Input: part model. Units: mm. Frame: model coordinates. A direction names the side the tool comes from. Give positions to 0.01 mm unless a question says otherwise; leave off trailing zeros. Loops run counter-clockwise (first coordinate to the right, second up) from the corner with the lowest first, then second, coordinate; pieces in that order, holes last. Notation, with made-up numbers: M -27,50 L -3,50 A21 ccw -3,55 Z; hole C 36,-15 d10. An arc over 180 degrees is marked long. Answer as a JSON object with one key per item and string values. Group by question number.
```python
from build123d import *

# Parameters (mm, degrees)
SKETCH_1_W           = 112
SKETCH_1_H           = 140
EXTRUDE_1_DEPTH      = 2.5
CUT_EXTRUDE_2_DEPTH  = 5
SKETCH_4_R           = 2.025
CUT_EXTRUDE_3_DEPTH  = 10
SKETCH_6_W           = 18
SKETCH_6_H           = 13
CUT_EXTRUDE_5_DEPTH  = 10
CUT_EXTRUDE_6_DEPTH  = 5
FILLET_1_R           = 3
SKETCH_8_R           = 1.525
CUT_EXTRUDE_7_DEPTH  = 5
SKETCH_10_R          = 2.525
CUT_EXTRUDE_9_DEPTH  = 40
FILLET_3_R           = 3
CUT_EXTRUDE_10_DEPTH = 78
EXTRUDE_2_DEPTH      = 5
EXTRUDE_3_DEPTH      = 5
FILLET_4_R           = 1.5
EXTRUDE_6_DEPTH      = 5
SKETCH_22_R          = 1.525
CUT_EXTRUDE_15_DEPTH = 5
SKETCH_24_R          = 2.025
CUT_EXTRUDE_17_DEPTH = 10


with BuildPart() as part:
    # 草图1 → 凸台-拉伸1 (new, symmetric)
    with BuildSketch(Plane.XY):
        Rectangle(SKETCH_1_W, SKETCH_1_H)
    extrude(amount=EXTRUDE_1_DEPTH, both=True)

    # 草图3 → 切除-拉伸2 (cut)
    with BuildSketch(Plane.XY.offset(2.5)):
        Polygon((-15, 70), (-56, 50), (-56, 70), align=None)
        Polygon((56, 70), (15, 70), (56, 50), align=None)
    extrude(amount=-CUT_EXTRUDE_2_DEPTH, mode=Mode.SUBTRACT)

    # 草图4 → 切除-拉伸3 (cut)
    with BuildSketch(Plane.XY.offset(2.5)):
        with Locations((0, -3.65)):
            Circle(SKETCH_4_R)
        with Locations((43, -3.65)):
            Circle(SKETCH_4_R)
        with Locations((-43, -3.65)):
            Circle(SKETCH_4_R)
        with Locations((-43, 23)):
            Circle(SKETCH_4_R)
        with Locations((0, 42.696305337)):
            Circle(SKETCH_4_R)
        with Locations((43, 23)):
            Circle(SKETCH_4_R)
    extrude(amount=-CUT_EXTRUDE_3_DEPTH, mode=Mode.SUBTRACT)

    # 草图6 → 切除-拉伸5 (cut)
    with BuildSketch(Plane(origin=(0, 0, -2.5), x_dir=(-1, 0, 0), z_dir=(0, 0, -1))):
        with Locations((47, -63.5)):
            Rectangle(SKETCH_6_W, SKETCH_6_H)
    cut_extrude_5 = extrude(amount=-CUT_EXTRUDE_5_DEPTH, mode=Mode.SUBTRACT)

    # 镜向2: 切除-拉伸5 across plane
    add(cut_extrude_5.mirror(Plane(origin=(0, 0, 0), x_dir=(0, 0, 1), z_dir=(1, 0, 0))), mode=Mode.SUBTRACT)

    # 草图7 → 切除-拉伸6 (cut)
    with BuildSketch(Plane.XY.offset(2.5)):
        Polygon((-3, 1.35), (-3, 35.822569262), (-38, 19.790692824), (-38, 1.35), align=None)
        Polygon((38, 19.790692824), (3, 35.822569262), (3, 1.35), (38, 1.35), align=None)
    extrude(amount=-CUT_EXTRUDE_6_DEPTH, mode=Mode.SUBTRACT)

    # 圆角1
    fillet_1_edges = [part.edges().sort_by_distance(p)[0] for p in [
        (-38, 19.790692824, 0),
        (-38, 1.35, 0),
        (-3, 1.35, 0),
        (-3, 35.822569262, 0),
        (3, 1.35, 0),
        (38, 1.35, 0),
        (38, 19.790692824, 0),
        (3, 35.822569262, 0),
    ]]
    fillet(fillet_1_edges, radius=FILLET_1_R)

    # 草图8 → 切除-拉伸7 (cut)
    with BuildSketch(Plane(origin=(0, 0, -2.5), x_dir=(-1, 0, 0), z_dir=(0, 0, -1))):
        with Locations((-53, 2)):
            Circle(SKETCH_8_R)
        with Locations((-53, -18)):
            Circle(SKETCH_8_R)
    cut_extrude_7 = extrude(amount=-CUT_EXTRUDE_7_DEPTH, mode=Mode.SUBTRACT)

    # 镜向3: 切除-拉伸7 across plane
    add(cut_extrude_7.mirror(Plane(origin=(0, 0, 0), x_dir=(0, 0, 1), z_dir=(1, 0, 0))), mode=Mode.SUBTRACT)

    # 草图10 → 切除-拉伸9 (cut)
    with BuildSketch(Plane.XY.offset(2.5)):
        with Locations((-30, -64)):
            Circle(SKETCH_10_R)
        with Locations((30, -64)):
            Circle(SKETCH_10_R)
    extrude(amount=-CUT_EXTRUDE_9_DEPTH, mode=Mode.SUBTRACT)

    # 圆角3
    fillet_3_edges = [part.edges().sort_by_distance(p)[0] for p in [
        (-56, 50, 0),
        (-15, 70, 0),
        (15, 70, 0),
        (56, 50, 0),
        (-56, -57, 0),
        (-38, -70, 0),
        (-38, -57, 0),
        (56, -57, 0),
        (38, -57, 0),
        (38, -70, 0),
    ]]
    fillet(fillet_3_edges, radius=FILLET_3_R)

    # 草图11 → 切除-拉伸10 (cut)
    with BuildSketch(Plane(origin=(0, 0, -2.5), x_dir=(-1, 0, 0), z_dir=(0, 0, -1))):
        Polygon((-6.884052732, -51), (-48, -11.425900755), (-48, -51), align=None)
        Polygon((-4, -8.65), (-45.115947268, -8.65), (-4, -48.224099245), align=None)
    cut_extrude_10 = extrude(amount=-CUT_EXTRUDE_10_DEPTH, mode=Mode.SUBTRACT)

    # 草图12 → 凸台-拉伸2 (add)
    with BuildSketch(Plane(origin=(0, 0, -2.5), x_dir=(-1, 0, 0), z_dir=(0, 0, -1))):
        Polygon((-27.442026366, -8.65), (-4, -31.212950377), (-2.613062807, -26.996075916), (-23.171036441, -7.209026293), align=None)
        Polygon((-49.386937193, -32.653924084), (-28.828963559, -52.440973707), (-24.557973634, -51), (-48, -28.437049623), align=None)
    extrude_2 = extrude(amount=-EXTRUDE_2_DEPTH)

    # 草图13 → 凸台-拉伸3 (add)
    with BuildSketch(Plane(origin=(0, 0, -2.5), x_dir=(-1, 0, 0), z_dir=(0, 0, -1))):
        Polygon((-29.446658669, -8.65), (-26.553352036, -51.135886105), (-22.553341331, -51), (-25.446647964, -8.514113895), align=None)
    extrude_3 = extrude(amount=-EXTRUDE_3_DEPTH)

    # 镜向5: 切除-拉伸10, 凸台-拉伸2, 凸台-拉伸3 across plane
    add(cut_extrude_10.mirror(Plane(origin=(0, 0, 0), x_dir=(0, 0, 1), z_dir=(1, 0, 0))), mode=Mode.SUBTRACT)
    add(extrude_2.mirror(Plane(origin=(0, 0, 0), x_dir=(0, 0, 1), z_dir=(1, 0, 0))))
    add(extrude_3.mirror(Plane(origin=(0, 0, 0), x_dir=(0, 0, 1), z_dir=(1, 0, 0))))

    # 圆角4
    fillet_4_edges = [part.edges().sort_by_distance(p)[0] for p in [
        (4, -48.224099245, 0),
        (45.115947268, -8.65, 0),
        (4, -8.65, 0),
        (6.884052732, -51, 0),
        (48, -51, 0),
        (48, -11.425900755, 0),
        (4, -25.661148868, 0),
        (21.673920902, -8.65, 0),
        (4, -31.212950377, 0),
        (48, -33.988851132, 0),
        (30.326079098, -51, 0),
        (48, -28.437049623, 0),
        (26.703219631, -48.935200727, 0),
        (25.296780369, -10.714799273, 0),
        (23.652453905, -34.860413872, 0),
        (27.942945899, -30.730815326, 0),
        (29.446658669, -8.65, 0),
        (24.057054101, -28.919184674, 0),
        (22.553341331, -51, 0),
        (28.347546095, -24.789586128, 0),
        (-45.115947268, -8.65, 0),
        (-4, -48.224099245, 0),
        (-4, -8.65, 0),
        (-48, -51, 0),
        (-6.884052732, -51, 0),
        (-48, -11.425900755, 0),
        (-21.673920902, -8.65, 0),
        (-4, -25.661148868, 0),
        (-4, -31.212950377, 0),
        (-48, -33.988851132, 0),
        (-30.326079098, -51, 0),
        (-48, -28.437049623, 0),
        (-26.703219631, -48.935200727, 0),
        (-25.296780369, -10.714799273, 0),
        (-23.652453905, -34.860413872, 0),
        (-24.057054101, -28.919184674, 0),
        (-22.553341331, -51, 0),
        (-27.942945899, -30.730815326, 0),
        (-28.347546095, -24.789586128, 0),
        (-29.446658669, -8.65, 0),
    ]]
    fillet(fillet_4_edges, radius=FILLET_4_R)

    # 草图21 → 凸台-拉伸6 (add)
    with BuildSketch(Plane(origin=(0, 0, -2.5), x_dir=(-1, 0, 0), z_dir=(0, 0, -1))):
        with BuildLine():
            Line((-20, -3), (-25.822161429, -3))
            Line((-25.822161429, -3), (-25.413558917, -9))
            Line((-25.413558917, -9), (-20, -9))
            ThreePointArc((-20, -9), (-17, -6), (-20, -3))
        make_face()
    extrude(amount=-EXTRUDE_6_DEPTH)

    # 草图22 → 切除-拉伸15 (cut)
    with BuildSketch(Plane(origin=(0, 0, -2.5), x_dir=(-1, 0, 0), z_dir=(0, 0, -1))):
        with Locations((0, -6)):
            Circle(SKETCH_22_R)
        with Locations((-20, -6)):
            Circle(SKETCH_22_R)
    extrude(amount=-CUT_EXTRUDE_15_DEPTH, mode=Mode.SUBTRACT)

    # 草图24 → 切除-拉伸17 (cut)
    with BuildSketch(Plane.XY.offset(2.5)):
        with Locations((-15, -64)):
            Circle(SKETCH_24_R)
        with Locations((15, -64)):
            Circle(SKETCH_24_R)
    extrude(amount=-CUT_EXTRUDE_17_DEPTH, mode=Mode.SUBTRACT)


solid = part.part
```
1. Material intervals for L1, parallel to X at y = 11.5, z = -0.9; L2, parallel to Y at x = -43, z = 0.65 (3 decimals); L3, parallel to Y at x = 39.5, z = 1, sorted ascending.
2. Mould query, pull axis Y, two halves, no side actions, for faces 3 (the flat face through (12, -8.65, 0)), 4 (the cylindrical face through (55.53, 49.74, -0.04)), 5 (the cylindrical face through (55.14, -56.1, 0.04)). Classes: pulls with the +Y half, pulls with the -Y half, needs draft (parallel to the pull), parting line crosses it, or undercut.
3. Section A-A (y = 6.5). Output: boundary loops of the cut face in (x, z), then the cut area to 3 significant figures.
4. Reachability of faces 1 (the flat face through (-1, 1, -2.5)), 2 (the flat face through (39.321, -42.343, -0.035)) from +Z, -Z, +X, -X, +Y, -Y: full face, straight path, thin tool, end or side. Return the list, or none.
5. Section B-B (y = 23). Output: boundary loops of the cut face in (x, z) (3 decimals).
6. Section D-D (z = 1.45). Count the separate pieces of the cut face and the enclosed holes in it, then the cut area to 3 significant figures.
7. First-contact query: P1, Ø1.5, axis at x = 19, z = 0.5, coming from the +Y side; P2, Ø1.5, axis at x = 39.5, z = -1.5, coming from the -Y side. Flat tips, straight axial feed; report the tip coordinate or a pass-through.
8. Section C-C (y = 53). Output: boundary loops of the cut face in (x, z), then the cut area to 4 significant figures.
Geometry results:
{
 "1": {"L1": "-56 to -38, -3 to 3, 38 to 56", "L2": "-57 to -51, -38.801 to -33.25, -16.238 to -5.675, -1.625 to 20.975, 25.025 to 56.341", "L3": "-57.4 to -51, -42.17 to -36.62, -19.61 to -14.06, -8.65 to 58.05"},
 "2": {"face 3": "undercut", "face 4": "pulls with the +Y half", "face 5": "pulls with the -Y half"},
 "3": {"outline": "M -56,-2.5 L -38,-2.5 L -38,2.5 L -56,2.5 Z; M -3,-2.5 L 3,-2.5 L 3,2.5 L -3,2.5 Z; M 38,-2.5 L 56,-2.5 L 56,2.5 L 38,2.5 Z", "area": "210 mm2"},
 "4": {"face 1": "-Z, +X, -X, +Y, -Y", "face 2": "+Z, -Z"},
 "5": {"outline": "M -56,-2.5 L -45.025,-2.5 L -45.025,2.5 L -56,2.5 Z; M -40.975,-2.5 L -30.994,-2.5 L -30.994,2.5 L -40.975,2.5 Z; M -3,-2.5 L 3,-2.5 L 3,2.5 L -3,2.5 Z; M 30.994,-2.5 L 40.975,-2.5 L 40.975,2.5 L 30.994,2.5 Z; M 45.025,-2.5 L 56,-2.5 L 56,2.5 L 45.025,2.5 Z"},
 "6": {"separate pieces": "1", "enclosed holes": "29", "area": "9,930 mm2"},
 "7": {"P1": "y = 68.41", "P2": "y = -58.02"},
 "8": {"outline": "M -49.85,-2.5 L 49.85,-2.5 L 49.85,2.5 L -49.85,2.5 Z", "area": "498.5 mm2"}
}
